```python
from build123d import *

# Parameters (mm, degrees)
SKETCH1_R                = 15
SKETCH1_R_2              = 7.5
BOSS_EXTRUDE1_DEPTH      = 210
BOSS_EXTRUDE1_DEPTH_BACK = 210
SKETCH3_R                = 3.1
CUT_EXTRUDE1_DEPTH       = 30


with BuildPart() as part:
    # Sketch1 → Boss-Extrude1 (new body, two sides)
    with BuildSketch(Plane.XY) as boss_extrude1_sk:
        Circle(SKETCH1_R)
        Circle(SKETCH1_R_2, mode=Mode.SUBTRACT)
    extrude(amount=BOSS_EXTRUDE1_DEPTH)
    extrude(boss_extrude1_sk.sketch, amount=-BOSS_EXTRUDE1_DEPTH_BACK)

    # Sketch3 → Cut-Extrude1 (cut)
    with BuildSketch(Plane(origin=(0, 0, 0), x_dir=(1, 0, 0), z_dir=(0, 1, 0))):
        with Locations((0, 195)):
            Circle(SKETCH3_R)
    cut_extrude1 = extrude(amount=CUT_EXTRUDE1_DEPTH, mode=Mode.SUBTRACT)

    # Mirror1: Cut-Extrude1 across plane
    add(cut_extrude1.mirror(Plane.XY), mode=Mode.SUBTRACT)


solid = part.part
```
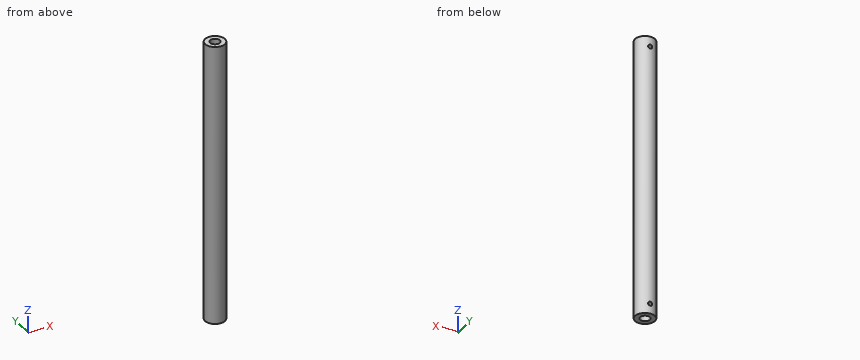
Work out the finished part from the listing and answer in its coordinate system (mm). Coordinates: 2 decimals unless noted, no trailing zeros. Order: outer loops, then holes, each group sorted by start corner. A loop starts at its lowest first (then second) coordinate and runs counter-clockwise, first axis right, second up. Notation, with made-up numbers: M -23,-5.5 L 5,-5.5 A18 cw 5,25.5 Z; hole C 85.5,15 d4. An arc over 180 degrees is marked long. Use CSV: the item, a comma, the result in double quotes.
1) Section C-C on x = -11 is taken. Write down the section's boundary in (y, z).
Worked out:
outline,"M -10.2,-210 L 10.2,-210 L 10.2,210 L -10.2,210 Z"
2) Section A-A on y = 0 is taken. Write down the section's boundary in (x, z).
Worked out:
outline,"M -15,-210 L -7.5,-210 L -7.5,210 L -15,210 Z; M 7.5,-210 L 15,-210 L 15,210 L 7.5,210 Z"
3) Flat-ended cylindrical pins translate along their axes: pin 1 Ø4 at (x, z) = (-10.5, -167) entering from +Y; pin 2 Ø1.5 at (y, z) = (-5.5, -134.5) entering from -X; pin 3 Ø10 at (y, z) = (-3, 106.5) entering from -X; pin 4 Ø4 at (x, z) = (-4, 32) entering from -Y. Find the tip coordinate at first contact, or state that the pin passes through.
Worked out:
pin 1,"stops at y = 12.36"
pin 2,"stops at x = -14.23"
pin 3,"stops at x = -15"
pin 4,"stops at y = -14.87"
4) Section B-B on z = 7 is taken. Write down the section's boundary in (x, y).
Worked out:
outline,"C 0,0 d30; hole C 0,0 d15"
5) Consider line 1 (Z direction, x = 0, y = 8.5); line 2 (X direction, y = 1, z = -179); line 3 (Y direction, x = 0, z = -124.5). Determine where each line is inside the solid, lowest interval first. Write a range as [from, to].
Worked out:
line 1,"z = [-210, -198.1], [-191.9, 191.9], [198.1, 210]"
line 2,"x = [-14.97, -7.43], [7.43, 14.97]"
line 3,"y = [-15, -7.5], [7.5, 15]"
